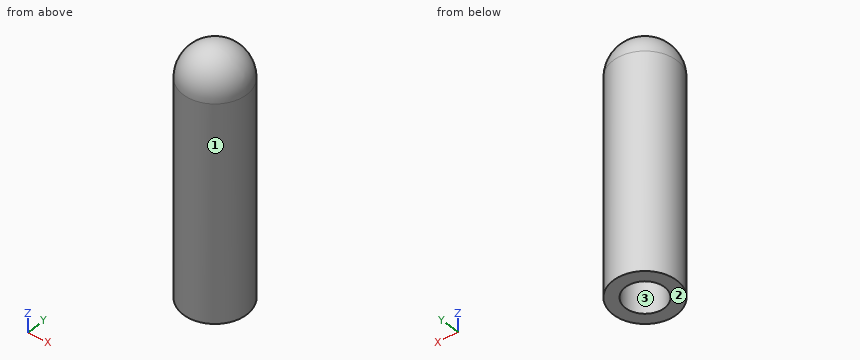
```python
from build123d import *

# Parameters (mm, degrees)
F0_R     = 2.794
F0_R_2   = 1.7145
F1_DEPTH = 21.971
F2_R     = 1.7145
F3_DEPTH = 1.778
F4_R     = 2.794


with BuildPart() as f1:
    # F0 (on Top) → F1 (new body)
    with BuildSketch(Plane.XY):
        Circle(F0_R)
        Circle(F0_R_2, mode=Mode.SUBTRACT)
    extrude(amount=F1_DEPTH)

    # F2 (on face) → F3 (join)
    with BuildSketch(Plane.XY.offset(21.971)):
        Circle(F2_R)
    extrude(amount=-F3_DEPTH)

    # F4
    f4_edges = [f1.edges().sort_by_distance(p)[0] for p in [
        (-2.794, 0, 21.971),
    ]]
    fillet(f4_edges, radius=F4_R)


solid = f1.part
```
CAD build for the part. Positions are in the model's coordinates, mm. Face numbers are marked on the shaded views. Coordinates: 2 decimals unless noted, no trailing zeros. Loops run counter-clockwise (first coordinate to the right, second up) from the corner with the lowest first, then second, coordinate; pieces in that order, holes last. Notation, with made-up numbers: (7.25, 51) - (51.25, 51) arc R16 cw to (51.25, 57) - close; hole circle Ø3 at (14, 64.25). An arc over 180 degrees is marked (long way). Use CSV: the item, a comma, the result in double quotes. Start each with the question number.
Q1. Probe probe 1 along Y at (x, z) = (0, 7.5); probe 2 along Y at (x, z) = (-0.55, 13); probe 3 along X at (y, z) = (-0.85, 5.75). List the from-to ranges inside material, lowest first. Write a range as from..to.
Q2. Two-plate mould, pull along X, no slides. Class the marked faces 1, 2 and 3: +X half, -X half, draft (parallel to the pull), parting line (faces both ways), or undercut.
Q3. Cut at A-A, the plane y = 0. List the corners of the cut face in (x, z), then the cut area to 3 significant figures.
Q4. Cut at D-D, the plane y = 2.35. List the corners of the cut face in (x, z).
Q5. Cut at C-C, the plane z = 2.5. List the corners of the cut face in (x, y).
Q6. Drop flat-ended pins along their axis: P1, Ø1, axis at x = -1.5, z = 6, coming from the -Y side; P2, Ø1.7, axis at x = -0.5, y = 0.5, coming from the -Z side. Give the stop position or say it passes through.
Here are the results:
1,probe 1,"-2.79..-1.71, 1.71..2.79"
1,probe 2,"-2.74..-1.62, 1.62..2.74"
1,probe 3,"-2.66..-1.49, 1.49..2.66"
2,face 1,"parting line"
2,face 2,"draft"
2,face 3,"undercut"
3,outline,"(-2.79, 0) - (-1.71, 0) - (-1.71, 20.19) - (1.71, 20.19) - (1.71, 0) - (2.79, 0) - (2.79, 19.18) arc R2.79 ccw to (-2.79, 19.18) - close"
3,area,"50.2 mm2"
4,outline,"(-1.51, 0) - (1.51, 0) - (1.51, 19.18) arc R1.51 ccw to (-1.51, 19.18) - close"
5,outline,"circle Ø5.59 at (0, 0); hole circle Ø3.43 at (0, 0)"
6,P1,"y = -2.61"
6,P2,"z = 20.19"
